from build123d import *

# Parameters (mm, degrees)
ESQUISSE1_R      = 2.5
ESQUISSE1_R_2    = 11
ESQUISSE1_R_3    = 2
EXTRUSION1_DEPTH = 3
CONG_1_R         = 10


with BuildPart() as part:
    # Esquisse1 → Extrusion1 (new body)
    with BuildSketch(Plane(origin=(0, 0, 0), x_dir=(1, 0, 0), z_dir=(0, 1, 0))):
        with BuildLine():
            Line((165, 0), (-165, 0))
            Line((-165, 0), (-165, -210))
            Line((-165, -210), (-149, -210))
            Line((-149, -210), (-132, -193))
            Line((-132, -193), (-132, -184))
            Line((-132, -184), (-100, -184))
            Line((-100, -184), (-63.363257782, -156.27367461))
            ThreePointArc((-63.363257782, -156.27367461), (0, -135), (63.363257782, -156.27367461))
            Line((63.363257782, -156.27367461), (100, -184))
            Line((100, -184), (132, -184))
            Line((132, -184), (132, -193))
            Line((132, -193), (149, -210))
            Line((149, -210), (165, -210))
            Line((165, -210), (165, 0))
        make_face()
        with Locations((-155, -10)):
            Circle(ESQUISSE1_R, mode=Mode.SUBTRACT)
        with Locations((155, -10)):
            Circle(ESQUISSE1_R, mode=Mode.SUBTRACT)
        with Locations((-155, -200)):
            Circle(ESQUISSE1_R, mode=Mode.SUBTRACT)
        with Locations((155, -200)):
            Circle(ESQUISSE1_R, mode=Mode.SUBTRACT)
        with Locations((-148, -172)):
            Circle(ESQUISSE1_R_2, mode=Mode.SUBTRACT)
        with Locations((-158.606601718, -161.393398282)):
            Circle(ESQUISSE1_R_3, mode=Mode.SUBTRACT)
        with Locations((-137.393398282, -161.393398282)):
            Circle(ESQUISSE1_R_3, mode=Mode.SUBTRACT)
        with Locations((-137.393398282, -182.606601718)):
            Circle(ESQUISSE1_R_3, mode=Mode.SUBTRACT)
        with Locations((-158.606601718, -182.606601718)):
            Circle(ESQUISSE1_R_3, mode=Mode.SUBTRACT)
        with Locations((148, -172)):
            Circle(ESQUISSE1_R_2, mode=Mode.SUBTRACT)
        with Locations((158.606601718, -182.606601718)):
            Circle(ESQUISSE1_R_3, mode=Mode.SUBTRACT)
        with Locations((137.393398282, -182.606601718)):
            Circle(ESQUISSE1_R_3, mode=Mode.SUBTRACT)
        with Locations((137.393398282, -161.393398282)):
            Circle(ESQUISSE1_R_3, mode=Mode.SUBTRACT)
        with Locations((158.606601718, -161.393398282)):
            Circle(ESQUISSE1_R_3, mode=Mode.SUBTRACT)
        with Locations((-155, -111)):
            Circle(ESQUISSE1_R, mode=Mode.SUBTRACT)
        with Locations((155, -111)):
            Circle(ESQUISSE1_R, mode=Mode.SUBTRACT)
        Polygon((-80.5, -26), (-115.5, -26), (-115.5, -12), (-144, -12), (-144, -111), (-115.5, -111), (-115.5, -97), (-80.5, -97), align=None, mode=Mode.SUBTRACT)
        Polygon((115.5, -26), (115.5, -12), (144, -12), (144, -111), (115.5, -111), (115.5, -97), (80.5, -97), (80.5, -26), align=None, mode=Mode.SUBTRACT)
        with BuildLine():
            Line((9.5, -27), (-9.5, -27))
            ThreePointArc((-9.5, -27), (-17, -34.5), (-9.5, -42))
            Line((-9.5, -42), (9.5, -42))
            ThreePointArc((9.5, -42), (17, -34.5), (9.5, -27))
        make_face(mode=Mode.SUBTRACT)
    extrude(amount=EXTRUSION1_DEPTH)

    # Congé1
    cong_1_edges = [part.edges().sort_by_distance(p)[0] for p in [
        (-165, 1.5, 0),
        (165, 1.5, 0),
        (165, 1.5, 210),
        (-165, 1.5, 210),
    ]]
    fillet(cong_1_edges, radius=CONG_1_R)


solid = part.part
Build history of the part. All positions in model axes, mm. A direction names the side the tool comes from. Coordinates: 2 decimals unless noted, no trailing zeros. Order: outer loops, then holes, each group sorted by start corner. A loop starts at its lowest first (then second) coordinate and runs counter-clockwise, first axis right, second up. Notation, with made-up numbers: (22, -15) - (55, -15) arc R12 ccw to (55, -5) - close; hole circle Ø7 at (-21.75, 41). An arc over 180 degrees is marked (long way). Write each question's results on one line, items separated by ' | '. Start each with the question number.
Item 1: Band-saw the part on D-D on x = 85. Write the cut outline in (y, z).
Item 2: Flat gauge pins, fed straight in: pin 1 (4.5 mm diameter, centred on x = -155, z = 111, fed in from -Y); pin 2 (1 mm diameter, centred on x = 53, y = 1.5, fed in from +Z). Where does each tip first touch, or does it go through?
Item 3: Band-saw the part on B-B on x = -106.5. Write the cut outline in (y, z).
Item 4: Wall check: probe 1 along X at (y, z) = (2.3, 25); probe 2 along X at (y, z) = (0.8, 55.5); probe 3 along X at (y, z) = (0.85, 169.5). Give the ranges that are in metal, low to high. Write a range as [from, to].
Item 5: Tool access for faces 4 (the face through (-81.9, 1.5, 170.3)), 5 (the face through (-162.15, 1.52, 206.99)), 6 (the face through (-17, 1.48, 34.34)): list every direction of +Z, -Z, +X, -X, +Y, -Y with a clear straight run to the whole face (end or side of a thin tool).
Item 6: Band-saw the part on C-C on z = 83.5. Write the cut outline in (x, y).
Item 7: Band-saw the part on A-A on z = 34.5. Write the cut outline in (x, y).
Item 8: Mould opens along X. For faces 1 (the face through (161.99, 1.52, 2.85)), 2 (the face through (-2, 3, 80)), 3 (the face through (-141, 1, 202)) say: released by +X, released by -X, zero draft, split by the parting line, or undercut.
Numbers:
1) outline: (0, 0) - (3, 0) - (3, 26) - (0, 26) - close; (0, 97) - (3, 97) - (3, 172.65) - (0, 172.65) - close
2) pin 1: through | pin 2: z = 149.65
3) outline: (0, 0) - (3, 0) - (3, 26) - (0, 26) - close; (0, 97) - (3, 97) - (3, 184) - (0, 184) - close
4) probe 1: [-165, -144], [-115.5, 115.5], [144, 165] | probe 2: [-165, -144], [-80.5, 80.5], [144, 165] | probe 3: [-165, -158.71], [-137.29, -80.84], [80.84, 137.29], [158.71, 165]
5) face 4: +Z, +Y, -Y | face 5: +Z, -X, +Y, -Y | face 6: +Y, -Y
6) outline: (-165, 0) - (-144, 0) - (-144, 3) - (-165, 3) - close; (-80.5, 0) - (80.5, 0) - (80.5, 3) - (-80.5, 3) - close; (144, 0) - (165, 0) - (165, 3) - (144, 3) - close
7) outline: (-165, 0) - (-144, 0) - (-144, 3) - (-165, 3) - close; (-80.5, 0) - (-17, 0) - (-17, 3) - (-80.5, 3) - close; (17, 0) - (80.5, 0) - (80.5, 3) - (17, 3) - close; (144, 0) - (165, 0) - (165, 3) - (144, 3) - close
8) face 1: released by +X | face 2: zero draft | face 3: undercut
